Build history of the part. All positions in model axes, mm. A direction names the side the tool comes from. Round coordinates to 2 decimals unless told otherwise and drop trailing zeros. Write each loop counter-clockwise with the first axis right and the second up, starting at its lowest first coordinate (ties: lowest second). Pieces come first, ordered by that corner, then holes. Notation, with made-up numbers: (3.25, 52.5) -> (32.25, 52.5) arc R18 ccw to (32.25, 85.5) -> close; hole circle Ø4 at (18.25, 52). An arc over 180 degrees is marked (long way). Return JSON: item names as keys, results as strings.
from build123d import *

# Parameters (mm, degrees)
ESQUISSE2_R                  = 8.5
ESQUISSE2_R_2                = 10
ENL_V_MAT_EXTRU_1_DEPTH      = 25
ESQUISSE3_R                  = 5
ENL_V_MAT_EXTRU_2_DEPTH      = 113.6
CONG_1_R                     = 2
ENL_V_MAT_EXTRU_3_DEPTH      = 5
ENL_V_MAT_EXTRU_3_DEPTH_BACK = 105.5
ESQUISSE4_R                  = 5


with BuildPart() as part:
    # Esquisse1 → Révolution1 (revolve)
    with BuildSketch(Plane.XY, mode=Mode.PRIVATE) as r_volution1_sk:
        Polygon((-75.054401386, 0), (199.945598614, 0), (199.945598614, 60), (189.945598614, 60), (189.945598614, 27.3), (-75.054401386, 27.3), align=None)
    revolve(r_volution1_sk.sketch.rotate(Axis((-75.054401386, 0, 0), (1, 0, 0)), 90), axis=Axis((-75.054401386, 0, 0), (1, 0, 0)))

    # Esquisse2 → Enlèv. mat.-Extru.1 (cut)
    with BuildSketch(Plane(origin=(199.945598614, 0, 0), x_dir=(0, 0, -1), z_dir=(1, 0, 0))):
        with Locations((0, 48)):
            Circle(ESQUISSE2_R)
        with Locations((0, -48)):
            Circle(ESQUISSE2_R)
        with Locations((-48, 0)):
            Circle(ESQUISSE2_R)
        with Locations((48, 0)):
            Circle(ESQUISSE2_R)
        Circle(ESQUISSE2_R_2)
    extrude(amount=-ENL_V_MAT_EXTRU_1_DEPTH, mode=Mode.SUBTRACT)

    # Esquisse3 → Enlèv. mat.-Extru.2 (cut)
    with BuildSketch(Plane(origin=(174.945598614, 0, 0), x_dir=(0, 0, -1), z_dir=(1, 0, 0))):
        Circle(ESQUISSE3_R)
    extrude(amount=-ENL_V_MAT_EXTRU_2_DEPTH, mode=Mode.SUBTRACT)

    # Congé1
    cong_1_edges = [part.edges().sort_by_distance(p)[0] for p in [
        (-75.054401386, 0, -27.3),
    ]]
    fillet(cong_1_edges, radius=CONG_1_R)

    # Esquisse4 → Enlèv. mat.-Extru.3 (cut, two sides: drawn at the far end of the back side and taken through both)
    with BuildSketch(Plane(origin=(0, 0, 0), x_dir=(1, 0, 0), z_dir=(0, 1, 0)).offset(-ENL_V_MAT_EXTRU_3_DEPTH_BACK)):
        with Locations(Location((59.445598614, 0, 0), (0, 0, 90))):
            Circle(ESQUISSE4_R)
    extrude(amount=ENL_V_MAT_EXTRU_3_DEPTH + ENL_V_MAT_EXTRU_3_DEPTH_BACK, mode=Mode.SUBTRACT)


solid = part.part
Q1. Wall check: L1, parallel to Y at x = 196.5, z = 0; L2, parallel to Y at x = 188.5, z = 0; L3, parallel to X at y = 24.5, z = -23.5. Give the ranges that are in metal, low to high.
Verdict:
{"L1": "y = -60 to -56.5, -39.5 to -10, 10 to 39.5, 56.5 to 60", "L2": "y = -27.3 to -10, 10 to 27.3", "L3": "x = 189.95 to 199.95"}
Q2. Two-plate mould, pull along X, no slides. Class faces 1 (the flat face through (-75.054, 0, 0)), 2 (the cylindrical face through (54.49, -11.38, 0.65)), 3 (the cylindrical face through (195.016, 55.167, -4.57)), 4 (the flat face through (199.946, -1, -12)): +X half, -X half, draft (parallel to the pull), parting line (faces both ways), or undercut.
Verdict:
{"face 1": "-X half", "face 2": "undercut", "face 3": "draft", "face 4": "+X half"}
Q3. 3-axis set-ups, long thin cutter, end or side, ignore diameter. For faces 5 (the cylindrical face through (195.016, 5.745, 54.265)), 6 (the flat face through (59, 5, 0)), 7 (the flat face through (174.946, -2, 5)), 8 (the flat face through (189.946, 26, 12)): which of +Z, -Z, +X, -X, +Y, -Y reach the whole face in a straight line?
Verdict:
{"face 5": "+X, -X", "face 6": "-Y", "face 7": "+X", "face 8": "-X"}
Q4. Pin check, flat tips, straight feed: pin 1 Ø3 at (y, z) = (38.5, 40.5) entering from -X; pin 2 Ø5 at (x, z) = (59, 2) entering from -Y; pin 3 Ø6 at (x, z) = (163, 5.5) entering from -Y. Stop position of each tip, or through.
Verdict:
{"pin 1": "stops at x = 189.95", "pin 2": "stops at y = 5", "pin 3": "stops at y = -27.19"}
Q5. Saw through at A-A on y = 48. List the corners of the cut face in (x, z), then the cut area to 3 significant figures.
Verdict:
{"outline": "(189.95, -36) -> (199.95, -36) -> (199.95, -8.5) -> (189.95, -8.5) -> close; (189.95, 8.5) -> (199.95, 8.5) -> (199.95, 36) -> (189.95, 36) -> close", "area": "550 mm²"}
Q6. Saw through at C-C on x = 127. List the corners of the cut face in (y, z), then the cut area to 3 significant figures.
Verdict:
{"outline": "circle Ø54.6 at (0, 0); hole circle Ø10 at (0, 0)", "area": "2,260 mm²"}
Q7. Saw through at D-D on x = 15. List the corners of the cut face in (y, z), then the cut area to 3 significant figures.
Verdict:
{"outline": "circle Ø54.6 at (0, 0)", "area": "2,340 mm²"}
